```python
from build123d import *

# Parameters (mm, degrees)
SKETCH5_R         = 25.4
STUB_DEPTH        = 67.5
CIRPATTERN1_COUNT = 3
CIRPATTERN1_ANGLE = 180
BORE_SKETCH_R     = 23.75
BORE_DEPTH        = 71
CIRPATTERN2_COUNT = 3
CIRPATTERN2_ANGLE = 180


with BuildPart() as part:
    # Sketch1 → Flange (revolve)
    with BuildSketch(Plane(origin=(0, 0, 0), x_dir=(0, 0, -1), z_dir=(1, 0, 0))):
        Polygon((-37.5, -70), (-37.5, -66.8), (-28.561202792, -64.9), (0, -64.9), (0, -67.5), (-26.1, -67.5), (-26.1, -70), align=None)
    revolve(axis=Axis((0, 0, 0), (0, -1, 0)))

    # Sketch5 → Stub (add)
    with BuildSketch(Plane.XZ.offset(67.5)):
        Circle(SKETCH5_R)
    extrude(amount=-STUB_DEPTH)


with BuildPart() as cirpattern1_1:
    # CirPattern1: pattern copy
    add(part.part.rotate(Axis((0, 0, 0), (0, 0, 1)), 1 * CIRPATTERN1_ANGLE / (CIRPATTERN1_COUNT - 1)))


with BuildPart() as cirpattern1_2:
    # CirPattern1: pattern copy
    add(part.part.rotate(Axis((0, 0, 0), (0, 0, 1)), 2 * CIRPATTERN1_ANGLE / (CIRPATTERN1_COUNT - 1)))


with BuildPart() as part_1:
    add(part.part)

    # Combine1: union CirPattern1_1, CirPattern1_2
    add(cirpattern1_1.part)
    add(cirpattern1_2.part)

    # Bore Sketch → Bore (cut, through all)
    with BuildSketch(Plane(origin=(0, 0, 0), x_dir=(1, 0, 0), z_dir=(0, 1, 0))):
        Circle(BORE_SKETCH_R)
    bore = extrude(amount=-BORE_DEPTH, mode=Mode.SUBTRACT)

    # CirPattern2: Bore ×3 about axis
    cirpattern2_axis = Axis((0, 0, -30.25), (0, 0, 1))
    for i in range(1, CIRPATTERN2_COUNT):
        add(bore.rotate(cirpattern2_axis, i * CIRPATTERN2_ANGLE / (CIRPATTERN2_COUNT - 1)), mode=Mode.SUBTRACT)


solid = part_1.part
```
Geometry check sheet. Reference: the model listing, model coordinates, mm. A direction names the side the tool comes from. Coordinates: 2 decimals unless noted, no trailing zeros. Order: outer loops, then holes, each group sorted by start corner. A loop starts at its lowest first (then second) coordinate and runs counter-clockwise, first axis right, second up. Notation, with made-up numbers: (-36.75, -20.5) - (-18.75, -20.5) arc R24 ccw to (-18.75, 11.5) - close; hole circle Ø10 at (-10, -19). An arc over 180 degrees is marked (long way). Answer as a JSON object with one key per item and string values. Group by question number.
Item 1: Sectioned sample at A-A, the plane y = 0. Record the cut outline in (x, z), and give its area (3 significant figures).
Item 2: Sectioned sample at B-B, the plane x = 62.5. Record the cut outline in (y, z).
Item 3: Tool access check on faces 1 (the face through (68.768, -17.64, -19.237)), 2 (the face through (-36.61, 68.38, -8.13)), 3 (the face through (64.992, 28.306, -6.286)). Record the directions out of +Z, -Z, +X, -X, +Y, -Y that give a thin tool (end or side, any length) a straight path to the whole face; none if there is none.
Item 4: Sectioned sample at C-C, the plane z = 0. Give the number of separate pieces and of enclosed holes in the cut face, and give its area (3 significant figures).
Item 5: Draft check along Z on faces 4 (the face through (-2, 64.9, -26)), 5 (the face through (67.5, 11.5, -21.1)), 6 (the face through (68.38, 36.61, -8.13)). Enter one of: +Z half, -Z half, draft (parallel to the pull), parting line (faces both ways), or undercut.
Item 6: Depth check by flat-ended pin: pin 1 Ø5 at (y, z) = (-10.5, -22.5) entering from -X; pin 2 Ø17 at (y, z) = (0.5, 13) entering from -X; pin 3 Ø4 at (y, z) = (15, 13.5) entering from -X. Enter the tip coordinate at first touch or a pass-through.
Item 7: Scan lines: probe 1 along Y at (x, z) = (59, -1); probe 2 along Y at (x, z) = (32.5, 12); probe 3 along Z at (x, y) = (68, 0). Record each from-to range of solid material in increasing order.
Resolved:
{
 "1": {"outline": "(0, -25.4) - (64.9, -25.4) - (64.9, -28.56) - (66.8, -37.5) - (70, -37.5) - (70, -26.1) - (67.5, -26.1) - (67.5, -23.75) - (0, -23.75) arc R23.75 cw to (0, 23.75) - (67.5, 23.75) - (67.5, 26.1) - (70, 26.1) - (70, 37.5) - (66.8, 37.5) - (64.9, 28.56) - (64.9, 25.4) - (0, 25.4) arc R25.4 ccw to start", "area": "453 mm^2"},
 "2": {"outline": "circle Ø50.8 at (0, 0); hole circle Ø47.5 at (0, 0)"},
 "3": {"face 1": "+X", "face 2": "+Y", "face 3": "none"},
 "4": {"separate pieces": "3", "enclosed holes": "0", "area": "815 mm^2"},
 "5": {"face 4": "draft", "face 5": "undercut", "face 6": "parting line"},
 "6": {"pin 1": "x = -15.66", "pin 2": "x = -25", "pin 3": "x = -22.65"},
 "7": {"probe 1": "-25.38 to -23.73, 23.73 to 25.38", "probe 2": "-70 to -66.19, -22.39 to -20.5, 20.5 to 22.39, 66.19 to 70", "probe 3": "-37.5 to -26.1, 26.1 to 37.5"}
}
